Part model, mm, in its own coordinate system. A direction names the side the tool comes from. Round coordinates to 2 decimals unless told otherwise and drop trailing zeros. Write each loop counter-clockwise with the first axis right and the second up, starting at its lowest first coordinate (ties: lowest second). Pieces come first, ordered by that corner, then holes.
1) Saw through at A-A on x = -5. Write the cut outline in (y, z).
2) Pull direction Y, two halves, no side cores. Call faces 6 (the flat face through (-11.3, 12.331, 25.7)), 7 (the flat face through (0, -6.669, 15)), 8 (the cylindrical face through (-10.082, 14.866, 27.165)): +Y half, -Y half, draft (parallel to the pull), parting line (faces both ways), or undercut.
3) Drill centre lines: L1, parallel to X at y = 1.35, z = 26.5; L2, parallel to Y at x = 5, z = 2; L3, parallel to X at y = 12.5, z = 27.5. Where is each one in solid material? Low to high.
4) Saw through at B-B on z = 26.5. Count the separate pieces of the cut face and the enclosed holes in it, and give its area (3 significant figures).
5) Flat gauge pins, fed straight in: pin 1 (12 mm diameter, centred on x = 1, z = 14.5, fed in from +Y); pin 2 (3 mm diameter, centred on x = 10, y = 11, fed in from -Z); pin 3 (1.7 mm diameter, centred on x = -10.43, z = 26.5, fed in from +Y); pin 4 (5 mm diameter, centred on y = 11, z = 14, fed in from +X). Where does each tip first touch, or does it go through?
6) Saw through at C-C on y = 3.25. Write the cut outline in (x, z).
7) Which spindle directions (+Z, -Z, +X, -X, +Y, -Y) get a long thin tool onto all of the face, cutting with end or side? Do faces 1 (the flat face through (-5, -4.669, 15)), 2 (the flat face through (0, 0.331, 10)), 3 (the flat face through (7.072, 1, 27)), 4 (the flat face through (0, 9, 23)), 5 (the flat face through (9, -1.669, 15)). Say none if no direction does.
8) Saw through at D-D on z = 11.5. Write the cut outline in (x, y), and give its area (3 significant figures).
```python
from build123d import *

# Parameters (mm, degrees)
EXTRUDE_1_DEPTH     = 30
FILLET_1_R          = 1.5
EXTRUDE_3_DEPTH     = 17
SKETCH_5_R          = 10.75
CUT_EXTRUDE_2_DEPTH = 29
SKETCH_6_W          = 7
SKETCH_6_H          = 7
SKETCH_6_R          = 0.75
EXTRUDE_4_DEPTH     = 2
EXTRUDE_START       = 15
SKETCH_8_W          = 7
SKETCH_8_H          = 7
SKETCH_8_R          = 0.75
EXTRUDE_5_DEPTH     = 5


with BuildPart() as part:
    # 草图1 → 凸台-拉伸1 (new body)
    with BuildSketch(Plane.XY):
        Polygon((-13.927970183, -1.669251604), (-4.090414819, -1.669251604), (-4.090414819, -4.669251604), (-7.590414819, -4.669251604), (-7.590414819, -6.669251604), (7.409585181, -6.669251604), (7.409585181, -4.669251604), (3.909585181, -4.669251604), (3.909585181, -1.669251604), (14.072029817, -1.669251604), (14.072029817, 0.330748396), (-13.927970183, 0.330748396), align=None)
    extrude(amount=EXTRUDE_1_DEPTH)

    # 圆角1
    fillet_1_edges = [part.edges().sort_by_distance(p)[0] for p in [
        (7.409585181, -4.669251604, 15),
        (-7.590414819, -4.669251604, 15),
    ]]
    fillet(fillet_1_edges, radius=FILLET_1_R)

    # 草图2 → 凸台-拉伸3 (add)
    with BuildSketch(Plane(origin=(0, 0.330748396, 0), x_dir=(1, 0, 0), z_dir=(0, 1, 0))):
        Polygon((-13.927970183, 0), (-12.427970183, 0), (-12.427970183, -21), (12.572029817, -21), (12.572029817, 0), (14.072029817, 0), (14.072029817, -21), (14.072029817, -23), (-13.927970183, -23), (-13.927970183, -21), align=None)
    extrude(amount=EXTRUDE_3_DEPTH)

    # 草图5 → 切除-拉伸2 (cut, through all)
    with BuildSketch(Plane.ZY.offset(13.927970183)):
        with Locations((11.5, 17.330748396)):
            Circle(SKETCH_5_R)
    extrude(amount=-CUT_EXTRUDE_2_DEPTH, mode=Mode.SUBTRACT)

    # 草图6 → 凸台-拉伸4 (add)
    with BuildSketch(Plane(origin=(0, 0.330748396, 0), x_dir=(1, 0, 0), z_dir=(0, 1, 0))):
        with Locations((-10.427970183, -26.5)):
            Rectangle(SKETCH_6_W, SKETCH_6_H)
        with Locations((-10.427970183, -26.5)):
            Circle(SKETCH_6_R, mode=Mode.SUBTRACT)
        with Locations((10.572029817, -26.5)):
            Rectangle(SKETCH_6_W, SKETCH_6_H)
        with Locations((10.572029817, -26.5)):
            Circle(SKETCH_6_R, mode=Mode.SUBTRACT)
    extrude(amount=EXTRUDE_4_DEPTH)

    # 草图8 → 凸台-拉伸5 (add)
    with BuildSketch(Plane(origin=(0, 2.330748396, 0), x_dir=(1, 0, 0), z_dir=(0, 1, 0)).offset(EXTRUDE_START)):
        with Locations((-10.427970183, -26.5)):
            Rectangle(SKETCH_8_W, SKETCH_8_H)
        with Locations((-10.427970183, -26.5)):
            Circle(SKETCH_8_R, mode=Mode.SUBTRACT)
        with Locations((10.572029817, -26.5)):
            Rectangle(SKETCH_8_W, SKETCH_8_H)
        with Locations((10.572029817, -26.5)):
            Circle(SKETCH_8_R, mode=Mode.SUBTRACT)
    extrude(amount=-EXTRUDE_5_DEPTH)


solid = part.part
```
Completed:
1. outline: (-6.67, 0) - (-4.67, 0) - (-4.67, 30) - (-6.67, 30) - close; (-1.67, 0) - (0.33, 0) - (0.33, 21) - (12.3, 21) arc R10.75 cw to (17.33, 22.25) - (17.33, 23) - (0.33, 23) - (0.33, 30) - (-1.67, 30) - close
2. face 6: undercut
2. face 7: -Y half
2. face 8: draft
3. L1: x = -13.93 to -11.18, -9.68 to -6.93, 7.07 to 9.82, 11.32 to 14.07
3. L2: y = -6.67 to -4.67, -1.67 to 0.33
3. L3: x = -13.93 to -6.93, 7.07 to 14.07
4. separate pieces: 5
4. enclosed holes: 0
4. area: 186 mm2
5. pin 1: stops at y = 0.33
5. pin 2: stops at z = 21
5. pin 3: stops at y = 17.33
5. pin 4: passes through
6. outline: (-13.93, 0) - (-12.43, 0) - (-12.43, 21) - (12.57, 21) - (12.57, 0) - (14.07, 0) - (14.07, 23) - (-13.93, 23) - close
7. face 1: +Z, -Z, -X
7. face 2: -Z, +Y
7. face 3: +Z, +Y
7. face 4: +Z
7. face 5: +Z, -Z, +X
8. outline: (-13.93, -1.67) - (-4.09, -1.67) - (-4.09, -4.67) - (-6.09, -4.67) arc R1.5 ccw to (-7.59, -6.17) - (-7.59, -6.67) - (7.41, -6.67) - (7.41, -6.17) arc R1.5 ccw to (5.91, -4.67) - (3.91, -4.67) - (3.91, -1.67) - (14.07, -1.67) - (14.07, 6.58) - (12.57, 6.58) - (12.57, 0.33) - (-12.43, 0.33) - (-12.43, 6.58) - (-13.93, 6.58) - close
8. area: 128 mm2
